CAD build for the part. Positions are in the model's coordinates, mm. Face numbers are marked on the shaded views. A direction names the side the tool comes from. Give positions to 0.01 mm unless a question says otherwise; leave off trailing zeros. Order: outer loops, then holes, each group sorted by start corner. A loop starts at its lowest first (then second) coordinate and runs counter-clockwise, first axis right, second up.
```python
from build123d import *

# Parameters (mm, degrees)
SKETCH1_W                = 9.525
SKETCH1_H                = 6.746875
CUT_EXTRUDE1_DEPTH       = 10.525
CUT_EXTRUDE2_DEPTH       = 10.525
CUT_EXTRUDE3_DEPTH       = 10.525
CUT_EXTRUDE4_DEPTH       = 10.525
CUT_EXTRUDE5_DEPTH       = 10.525
CUT_EXTRUDE6_DEPTH       = 10.525
CUT_EXTRUDE7_DEPTH       = 10.525
CUT_EXTRUDE8_DEPTH       = 10.525
CUT_EXTRUDE9_DEPTH       = 10.525
CUT_EXTRUDE10_DEPTH      = 10.525
CUT_EXTRUDE11_DEPTH      = 10.525
CUT_EXTRUDE12_DEPTH      = 10.525
CUT_EXTRUDE13_DEPTH      = 10.525
CUT_EXTRUDE14_DEPTH      = 10.525
CUT_EXTRUDE15_DEPTH      = 10.525
SKETCH17_R               = 4.7625
BOSS_EXTRUDE1_DEPTH      = 7.1755
SKETCH18_W               = 6.35
SKETCH18_H               = 6.35
BOSS_EXTRUDE2_DEPTH      = 13.0175
M3_CLEARANCE_HOLE1_D     = 3.4544
M3_CLEARANCE_HOLE1_DEPTH = 16.93164
M3_CLEARANCE_HOLE1_TIP   = 1.037806461


with BuildPart() as part:
    # Sketch1 → Revolve1 (revolve)
    with BuildSketch(Plane(origin=(0, 0, 0), x_dir=(-1, 0, 0), z_dir=(0, 0, -1))):
        with Locations((-1.5875, 3.3734375)):
            Rectangle(SKETCH1_W, SKETCH1_H)
    revolve(axis=Axis((6.35, 0, 0), (-1, 0, 0)))

    # Sketch2 → Cut-Extrude1 (cut, through all)
    with BuildSketch(Plane(origin=(6.35, 0, 0), x_dir=(0, 0, -1), z_dir=(1, 0, 0))):
        with BuildLine():
            ThreePointArc((-4.893369276, -4.644917588), (-3.965713624, -5.458336534), (-2.905444874, -6.089229208))
            ThreePointArc((-2.905444874, -6.089229208), (-2.92382812, -5.1271904), (-2.559987212, -4.236417473))
            ThreePointArc((-2.559987212, -4.236417473), (-2.909434136, -4.004492544), (-3.23799289, -3.743817514))
            ThreePointArc((-3.23799289, -3.743817514), (-3.972735262, -4.365114753), (-4.893369276, -4.644917588))
        make_face()
    extrude(amount=-CUT_EXTRUDE1_DEPTH, mode=Mode.SUBTRACT)

    # Sketch3 → Cut-Extrude2 (cut, through all)
    with BuildSketch(Plane(origin=(6.35, 0, 0), x_dir=(0, 0, -1), z_dir=(1, 0, 0))):
        with BuildLine():
            ThreePointArc((-6.359573461, -2.253030771), (-5.842965146, -3.3734375), (-5.130968614, -4.381036789))
            ThreePointArc((-5.130968614, -4.381036789), (-4.75646611, -3.494693465), (-4.061770911, -2.828919335))
            ThreePointArc((-4.061770911, -2.828919335), (-4.286674194, -2.4749125), (-4.480801464, -2.103137126))
            ThreePointArc((-4.480801464, -2.103137126), (-5.404726374, -2.37187375), (-6.359573461, -2.253030771))
        make_face()
    extrude(amount=-CUT_EXTRUDE2_DEPTH, mode=Mode.SUBTRACT)

    # Sketch4 → Cut-Extrude3 (cut, through all)
    with BuildSketch(Plane(origin=(6.35, 0, 0), x_dir=(0, 0, -1), z_dir=(1, 0, 0))):
        with BuildLine():
            ThreePointArc((-6.726149621, 0.528425534), (-6.709914913, -0.705240476), (-6.469301267, -1.915323309))
            ThreePointArc((-6.469301267, -1.915323309), (-5.766667898, -1.257932283), (-4.861237519, -0.932275343))
            ThreePointArc((-4.861237519, -0.932275343), (-4.922709341, -0.517397601), (-4.948838759, -0.098805222))
            ThreePointArc((-4.948838759, -0.098805222), (-5.902191196, 0.031485771), (-6.726149621, 0.528425534))
        make_face()
    extrude(amount=-CUT_EXTRUDE3_DEPTH, mode=Mode.SUBTRACT)

    # Sketch5 → Cut-Extrude4 (cut, through all)
    with BuildSketch(Plane(origin=(6.35, 0, 0), x_dir=(0, 0, -1), z_dir=(1, 0, 0))):
        with BuildLine():
            ThreePointArc((-5.929713406, 3.218512264), (-6.416659433, 2.084899034), (-6.68903296, 0.881566972))
            ThreePointArc((-6.68903296, 0.881566972), (-5.779760418, 1.196336819), (-4.820151997, 1.125567525))
            ThreePointArc((-4.820151997, 1.125567525), (-4.707563321, 1.529580044), (-4.561176873, 1.922611002))
            ThreePointArc((-4.561176873, 1.922611002), (-5.37911354, 2.429401117), (-5.929713406, 3.218512264))
        make_face()
    extrude(amount=-CUT_EXTRUDE4_DEPTH, mode=Mode.SUBTRACT)

    # Sketch6 → Cut-Extrude5 (cut, through all)
    with BuildSketch(Plane(origin=(6.35, 0, 0), x_dir=(0, 0, -1), z_dir=(1, 0, 0))):
        with BuildLine():
            ThreePointArc((-5.752170086, 3.526026314), (-4.793479854, 3.443748417), (-3.945618406, 2.988789542))
            ThreePointArc((-3.945618406, 2.988789542), (-3.678436836, 3.312079404), (-3.384846069, 3.611590317))
            ThreePointArc((-3.384846069, 3.611590317), (-3.925938286, 4.40725094), (-4.107975873, 5.352088984))
            ThreePointArc((-4.107975873, 5.352088984), (-5.013905244, 4.51454056), (-5.752170086, 3.526026314))
        make_face()
    extrude(amount=-CUT_EXTRUDE5_DEPTH, mode=Mode.SUBTRACT)

    # Sketch7 → Cut-Extrude6 (cut, through all)
    with BuildSketch(Plane(origin=(6.35, 0, 0), x_dir=(0, 0, -1), z_dir=(1, 0, 0))):
        with BuildLine():
            ThreePointArc((-3.820704747, 5.560803674), (-2.978363076, 5.095704628), (-2.388851547, 4.335222695))
            ThreePointArc((-2.388851547, 4.335222695), (-2.013275204, 4.521890145), (-1.623244629, 4.676092857))
            ThreePointArc((-1.623244629, 4.676092857), (-1.793932636, 5.623047036), (-1.575931992, 6.560240897))
            ThreePointArc((-1.575931992, 6.560240897), (-2.744201289, 6.16357701), (-3.820704747, 5.560803674))
        make_face()
    extrude(amount=-CUT_EXTRUDE6_DEPTH, mode=Mode.SUBTRACT)

    # Sketch8 → Cut-Extrude7 (cut, through all)
    with BuildSketch(Plane(origin=(6.35, 0, 0), x_dir=(0, 0, -1), z_dir=(1, 0, 0))):
        with BuildLine():
            ThreePointArc((1.228604847, 6.63406756), (0, 6.746875), (-1.228604847, 6.63406756))
            ThreePointArc((-1.228604847, 6.63406756), (-0.648260265, 5.866567216), (-0.419030554, 4.93205646))
            ThreePointArc((-0.419030554, 4.93205646), (0, 4.949825), (0.419030554, 4.93205646))
            ThreePointArc((0.419030554, 4.93205646), (0.648260265, 5.866567216), (1.228604847, 6.63406756))
        make_face()
    extrude(amount=-CUT_EXTRUDE7_DEPTH, mode=Mode.SUBTRACT)

    # Sketch9 → Cut-Extrude8 (cut, through all)
    with BuildSketch(Plane(origin=(6.35, 0, 0), x_dir=(0, 0, -1), z_dir=(1, 0, 0))):
        with BuildLine():
            ThreePointArc((3.820704747, 5.560803674), (2.744201289, 6.16357701), (1.575931992, 6.560240897))
            ThreePointArc((1.575931992, 6.560240897), (1.793932636, 5.623047036), (1.623244629, 4.676092857))
            ThreePointArc((1.623244629, 4.676092857), (2.013275204, 4.521890145), (2.388851547, 4.335222695))
            ThreePointArc((2.388851547, 4.335222695), (2.978363076, 5.095704628), (3.820704747, 5.560803674))
        make_face()
    extrude(amount=-CUT_EXTRUDE8_DEPTH, mode=Mode.SUBTRACT)

    # Sketch10 → Cut-Extrude9 (cut, through all)
    with BuildSketch(Plane(origin=(6.35, 0, 0), x_dir=(0, 0, -1), z_dir=(1, 0, 0))):
        with BuildLine():
            ThreePointArc((5.752170086, 3.526026314), (5.013905244, 4.51454056), (4.107975873, 5.352088984))
            ThreePointArc((4.107975873, 5.352088984), (3.925938286, 4.40725094), (3.384846069, 3.611590317))
            ThreePointArc((3.384846069, 3.611590317), (3.678436836, 3.312079404), (3.945618406, 2.988789542))
            ThreePointArc((3.945618406, 2.988789542), (4.793479854, 3.443748417), (5.752170086, 3.526026314))
        make_face()
    extrude(amount=-CUT_EXTRUDE9_DEPTH, mode=Mode.SUBTRACT)

    # Sketch11 → Cut-Extrude10 (cut, through all)
    with BuildSketch(Plane(origin=(6.35, 0, 0), x_dir=(0, 0, -1), z_dir=(1, 0, 0))):
        with BuildLine():
            ThreePointArc((6.68903296, 0.881566972), (6.416659433, 2.084899034), (5.929713406, 3.218512264))
            ThreePointArc((5.929713406, 3.218512264), (5.37911354, 2.429401117), (4.561176873, 1.922611002))
            ThreePointArc((4.561176873, 1.922611002), (4.707563321, 1.529580044), (4.820151997, 1.125567525))
            ThreePointArc((4.820151997, 1.125567525), (5.779760418, 1.196336819), (6.68903296, 0.881566972))
        make_face()
    extrude(amount=-CUT_EXTRUDE10_DEPTH, mode=Mode.SUBTRACT)

    # Sketch12 → Cut-Extrude11 (cut, through all)
    with BuildSketch(Plane(origin=(6.35, 0, 0), x_dir=(0, 0, -1), z_dir=(1, 0, 0))):
        with BuildLine():
            ThreePointArc((6.469301267, -1.915323309), (6.709914913, -0.705240476), (6.726149621, 0.528425534))
            ThreePointArc((6.726149621, 0.528425534), (5.902191196, 0.031485771), (4.948838759, -0.098805222))
            ThreePointArc((4.948838759, -0.098805222), (4.922709341, -0.517397601), (4.861237519, -0.932275343))
            ThreePointArc((4.861237519, -0.932275343), (5.766667898, -1.257932283), (6.469301267, -1.915323309))
        make_face()
    extrude(amount=-CUT_EXTRUDE11_DEPTH, mode=Mode.SUBTRACT)

    # Sketch13 → Cut-Extrude12 (cut, through all)
    with BuildSketch(Plane(origin=(6.35, 0, 0), x_dir=(0, 0, -1), z_dir=(1, 0, 0))):
        with BuildLine():
            ThreePointArc((5.130968614, -4.381036789), (5.842965146, -3.3734375), (6.359573461, -2.253030771))
            ThreePointArc((6.359573461, -2.253030771), (5.404726374, -2.37187375), (4.480801464, -2.103137126))
            ThreePointArc((4.480801464, -2.103137126), (4.286674194, -2.4749125), (4.061770911, -2.828919335))
            ThreePointArc((4.061770911, -2.828919335), (4.75646611, -3.494693465), (5.130968614, -4.381036789))
        make_face()
    extrude(amount=-CUT_EXTRUDE12_DEPTH, mode=Mode.SUBTRACT)

    # Sketch14 → Cut-Extrude13 (cut, through all)
    with BuildSketch(Plane(origin=(6.35, 0, 0), x_dir=(0, 0, -1), z_dir=(1, 0, 0))):
        with BuildLine():
            ThreePointArc((2.905444874, -6.089229208), (3.965713624, -5.458336534), (4.893369276, -4.644917588))
            ThreePointArc((4.893369276, -4.644917588), (3.972735262, -4.365114753), (3.23799289, -3.743817514))
            ThreePointArc((3.23799289, -3.743817514), (2.909434136, -4.004492544), (2.559987212, -4.236417473))
            ThreePointArc((2.559987212, -4.236417473), (2.92382812, -5.1271904), (2.905444874, -6.089229208))
        make_face()
    extrude(amount=-CUT_EXTRUDE13_DEPTH, mode=Mode.SUBTRACT)

    # Sketch15 → Cut-Extrude14 (cut, through all)
    with BuildSketch(Plane(origin=(6.35, 0, 0), x_dir=(0, 0, -1), z_dir=(1, 0, 0))):
        with BuildLine():
            ThreePointArc((0.17754332, -6.744538578), (1.402754189, -6.599439594), (2.581057087, -6.233655956))
            ThreePointArc((2.581057087, -6.233655956), (1.853822132, -5.603587759), (1.435305929, -4.737157842))
            ThreePointArc((1.435305929, -4.737157842), (1.029126485, -4.841659448), (0.615558467, -4.911400544))
            ThreePointArc((0.615558467, -4.911400544), (0.585633687, -5.873149535), (0.17754332, -6.744538578))
        make_face()
    extrude(amount=-CUT_EXTRUDE14_DEPTH, mode=Mode.SUBTRACT)

    # Sketch16 → Cut-Extrude15 (cut, through all)
    with BuildSketch(Plane(origin=(6.35, 0, 0), x_dir=(0, 0, -1), z_dir=(1, 0, 0))):
        with BuildLine():
            ThreePointArc((-2.581057087, -6.233655956), (-1.402754189, -6.599439594), (-0.17754332, -6.744538578))
            ThreePointArc((-0.17754332, -6.744538578), (-0.585633687, -5.873149535), (-0.615558467, -4.911400544))
            ThreePointArc((-0.615558467, -4.911400544), (-1.029126485, -4.841659448), (-1.435305929, -4.737157842))
            ThreePointArc((-1.435305929, -4.737157842), (-1.853822132, -5.603587759), (-2.581057087, -6.233655956))
        make_face()
    extrude(amount=-CUT_EXTRUDE15_DEPTH, mode=Mode.SUBTRACT)

    # Sketch17 → Boss-Extrude1 (add)
    with BuildSketch(Plane(origin=(6.35, 0, 0), x_dir=(0, 0, -1), z_dir=(1, 0, 0))):
        Circle(SKETCH17_R)
    extrude(amount=BOSS_EXTRUDE1_DEPTH)

    # Sketch18 → Boss-Extrude2 (add)
    with BuildSketch(Plane(origin=(13.5255, 0, 0), x_dir=(0, 0, -1), z_dir=(1, 0, 0))):
        Rectangle(SKETCH18_W, SKETCH18_H)
    extrude(amount=BOSS_EXTRUDE2_DEPTH)

    # M3 Clearance Hole1
    with Locations(Plane(origin=(26.543, 0, 0), x_dir=(0, 0, -1), z_dir=(1, 0, 0))):
        with Locations((0, 0)):
            Hole(M3_CLEARANCE_HOLE1_D / 2, depth=M3_CLEARANCE_HOLE1_DEPTH)
            with Locations((0, 0, -(M3_CLEARANCE_HOLE1_DEPTH + M3_CLEARANCE_HOLE1_TIP / 2))):  # 118° drill point
                Cone(0, M3_CLEARANCE_HOLE1_D / 2, M3_CLEARANCE_HOLE1_TIP, mode=Mode.SUBTRACT)


solid = part.part
```
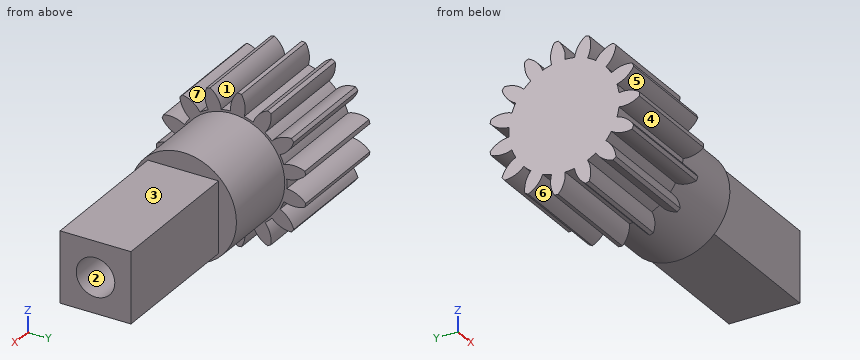
Item 1: Slice it at A-A (x = 20.25). Give the cut face in (y, z) (3 decimals).
Item 2: Two-plate mould, pull along Z, no slides. Class the marked faces 5, 6 and 7: released by +Z, released by -Z, zero draft, split by the parting line, or undercut.
Item 3: Tool access for the marked faces 1, 2, 3 and 4: list every direction of +Z, -Z, +X, -X, +Y, -Y with a clear straight run to the whole face (end or side of a thin tool).
Item 4: Slice it at C-C (x = 12). Give the cut face in (y, z) (1 decimal).
Item 5: Wall check: L1, parallel to Y at x = 15.5, z = 0 (3 decimals); L2, parallel to Y at x = 3.75, z = -5.5. Give the ranges that are in metal, low to high.
Item 6: Drop flat-ended pins along their axis: pin 1 Ø1 at (x, y) = (19, -1.5) entering from +Z (3 decimals); pin 2 Ø1.5 at (y, z) = (5, -4) entering from +X; pin 3 Ø2 at (x, z) = (20.5, 2) entering from -Y (3 decimals); pin 4 Ø2 at (x, z) = (20.5, -5) entering from +Y. Give the stop position or say it passes through.
A:
1. outline: (-3.175, -3.175) - (3.175, -3.175) - (3.175, 3.175) - (-3.175, 3.175) - close; hole circle Ø3.454 at (0, 0)
2. face 5: undercut
2. face 6: released by -Z
2. face 7: released by +Z
3. face 1: +Z, +X, -X
3. face 2: +X
3. face 3: +Z, +X, +Y, -Y
3. face 4: +X, -X
4. outline: circle Ø9.5 at (0, 0); hole circle Ø3.5 at (0, 0)
5. L1: y = -3.175 to -1.727, 1.727 to 3.175
5. L2: y = -2.38 to -1.12, -0.07 to 1.22, 2.55 to 3.54
6. pin 1: stops at z = 3.175
6. pin 2: stops at x = 6.35
6. pin 3: stops at y = -3.175
6. pin 4: passes through
